Geometry: final body of the model. Coordinates: model frame, mm. A direction names the side the tool comes from. Round coordinates to 2 decimals unless told otherwise and drop trailing zeros. Loops run counter-clockwise (first coordinate to the right, second up) from the corner with the lowest first, then second, coordinate; pieces in that order, holes last. Notation, with made-up numbers: (30.25, -17.75) - (79.25, -17.75) arc R19 ccw to (79.25, 6.25) - close; hole circle Ø3 at (-6.75, -21). An arc over 180 degrees is marked (long way). Write item = value, one per line. Start each with the question number.
Item 1: Draft query along Y for faces 3 (the cylindrical face through (-14.35, 11.62, 2.96)), 4 (the flat face through (-33.782, 2, 3)), 5 (the flat face through (-15.582, 2, 4)), 6 (the flat face through (-24, 10.425, 4)). Return one class per face: pulls with the +Y half, pulls with the -Y half, needs draft (parallel to the pull), parting line crosses it, or undercut.
Item 2: Section D-D (x = -30.25). Return loops of the section in (y, z), plus the area to 3 significant figures.
Item 3: Line query: line 1 (Y direction, x = -20.5, z = 4.6); line 2 (X direction, y = -2.75, z = 3.7); line 3 (Z direction, x = -17.5, y = -2.75). Output: solid intervals per line, ascending. Write a range as from..to.
Item 4: Section C-C (x = -24.75). Return loops of the section in (y, z).
Item 5: Section A-A (y = -3). Return loops of the section in (x, z).
Item 6: Access query for faces 1 (the flat face through (-33, 2, 6)), 2 (the flat face through (-24, -5.975, 4)). Directions: +Z, -Z, +X, -X, +Y, -Y. A direction counts if a zero-diameter tool reaches every point of the face in a straight line with its end or side. Return the directions, or none.
Item 7: First-contact query: pin 1 (6.5 mm diameter, centred on x = -23.78, y = 2.23, fed in from +Z); pin 2 (5 mm diameter, centred on x = -18, y = 4, fed in from +Z). Flat tips, straight axial feed; report the tip coordinate or a pass-through.
Item 8: Section B-B (z = 4.35). Return loops of the section in (x, y), plus the area to 3 significant figures.
from build123d import *

# Parameters (mm, degrees)
F1_DEPTH = 2
F2_W     = 16.4
F2_H     = 16.4
F3_DEPTH = 4
F4_R     = 2.5
F5_DEPTH = 25


with BuildPart() as f1:
    # F0 (on Top) → F1 (new body)
    with BuildSketch(Plane.XY):
        with BuildLine():
            Line((-15.782069, 12.225087), (-31.782069, 12.225087))
            ThreePointArc((-31.782069, 12.225087), (-33.196283, 11.6393), (-33.782069, 10.225087))
            Line((-33.782069, 10.225087), (-33.782069, -5.774913))
            ThreePointArc((-33.782069, -5.774913), (-33.196283, -7.189127), (-31.782069, -7.774913))
            Line((-31.782069, -7.774913), (-15.782069, -7.774913))
            ThreePointArc((-15.782069, -7.774913), (-14.367856, -7.189127), (-13.782069, -5.774913))
            Line((-13.782069, -5.774913), (-13.782069, 10.225087))
            ThreePointArc((-13.782069, 10.225087), (-14.367856, 11.6393), (-15.782069, 12.225087))
        make_face()
    extrude(amount=F1_DEPTH)

    # F2 (on face) → F3 (join)
    with BuildSketch(Plane.XY.offset(2)):
        with BuildLine():
            ThreePointArc((-13.782069, 10.225087), (-14.367856, 11.6393), (-15.782069, 12.225087))
            Line((-15.782069, 12.225087), (-31.782069, 12.225087))
            ThreePointArc((-31.782069, 12.225087), (-33.196283, 11.6393), (-33.782069, 10.225087))
            Line((-33.782069, 10.225087), (-33.782069, -5.774913))
            ThreePointArc((-33.782069, -5.774913), (-33.196283, -7.189127), (-31.782069, -7.774913))
            Line((-31.782069, -7.774913), (-15.782069, -7.774913))
            ThreePointArc((-15.782069, -7.774913), (-14.367856, -7.189127), (-13.782069, -5.774913))
            Line((-13.782069, -5.774913), (-13.782069, 10.225087))
        make_face()
        with Locations((-23.782069, 2.225087)):
            Rectangle(F2_W, F2_H, mode=Mode.SUBTRACT)
    extrude(amount=F3_DEPTH)

    # F4 (on face) → F5 (cut)
    with BuildSketch(Plane.XY.offset(2)):
        with Locations((-23.782069, 2.225087)):
            Circle(F4_R)
    extrude(amount=-F5_DEPTH, mode=Mode.SUBTRACT)


solid = f1.part
Taken from the geometry:
q1.face_3 = pulls with the +Y half
q1.face_4 = needs draft
q1.face_5 = undercut
q1.face_6 = undercut
q2.outline = (-7.77, 0) - (12.23, 0) - (12.23, 6) - (10.43, 6) - (10.43, 2) - (-5.97, 2) - (-5.97, 6) - (-7.77, 6) - close
q2.area = 54.4 mm^2
q3.line_1 = -7.77..-5.97, 10.43..12.23
q3.line_2 = -33.78..-31.98, -15.58..-13.78
q3.line_3 = 0..2
q4.outline = (-7.77, 0) - (-0.08, 0) - (-0.08, 2) - (-5.97, 2) - (-5.97, 6) - (-7.77, 6) - close; (4.53, 0) - (12.23, 0) - (12.23, 6) - (10.43, 6) - (10.43, 2) - (4.53, 2) - close
q5.outline = (-33.78, 0) - (-13.78, 0) - (-13.78, 6) - (-15.58, 6) - (-15.58, 2) - (-31.98, 2) - (-31.98, 6) - (-33.78, 6) - close
q6.face_1 = +Z, +X, -X, +Y, -Y
q6.face_2 = +Z
q7.pin_1 = 2
q7.pin_2 = 6
q8.outline = (-33.78, -5.77) arc R2 ccw to (-31.78, -7.77) - (-15.78, -7.77) arc R2 ccw to (-13.78, -5.77) - (-13.78, 10.23) arc R2 ccw to (-15.78, 12.23) - (-31.78, 12.23) arc R2 ccw to (-33.78, 10.23) - close; hole (-31.98, -5.97) - (-15.58, -5.97) - (-15.58, 10.43) - (-31.98, 10.43) - close
q8.area = 128 mm^2
